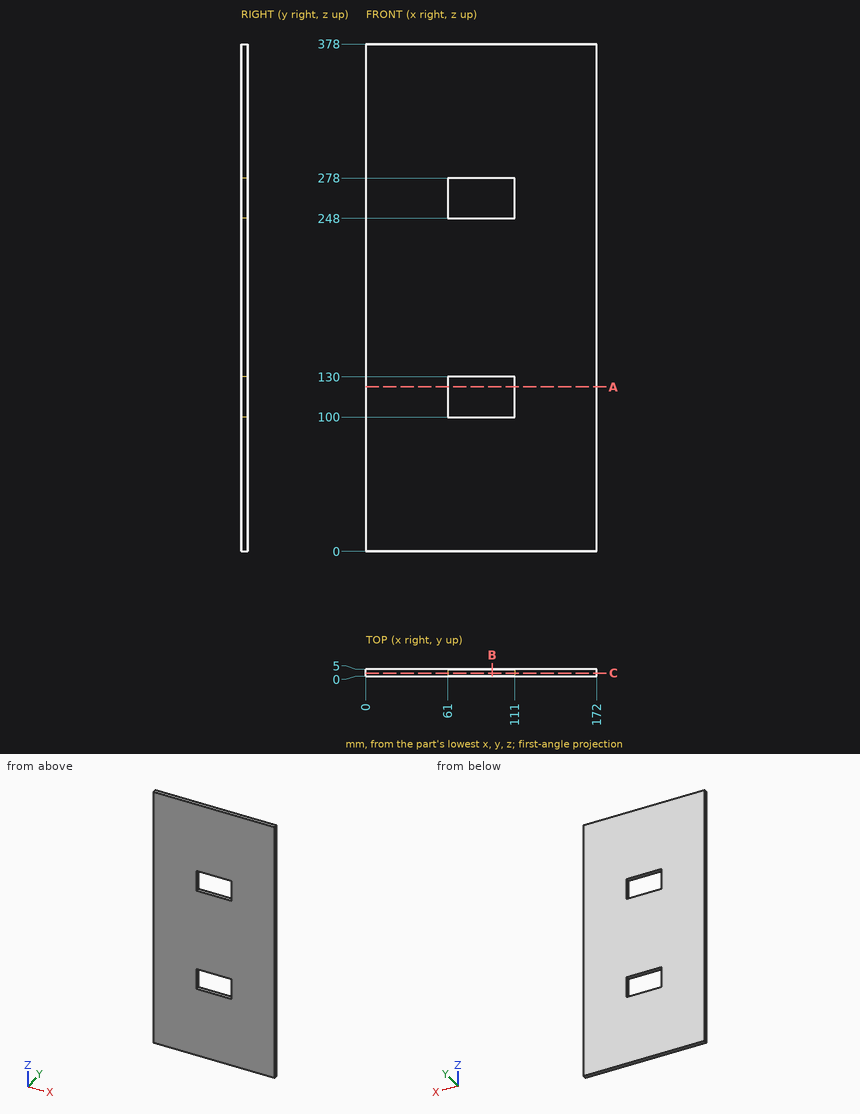
Source: three-view drawing plus pictorial views. Frame: mm from the lowest corner of the part. Round coordinates to 2 decimals unless told otherwise and drop trailing zeros. Order: outer loops, then holes, each group sorted by start corner. A loop starts at its lowest first (then second) coordinate and runs counter-clockwise, first axis right, second up. Notation, with made-up numbers: M 30,-6.5 L 89,-6.5 A28 ccw 89,22.5 Z; hole C -38,31 d1. An arc over 180 degrees is marked long. One line per item, written item: value.
(1) Pin query (flat end, axial travel): P1, Ø1.5, axis at x = 35.5, y = 2, coming from the -Z side. Return the tip coordinate at first contact, or that it passes through.
Result sheet:
P1: z = 0
(2) Cut plane B-B (x = 94). Return the cut outline in (y, z).
Result sheet:
outline: M 0,0 L 5,0 L 5,100 L 0,100 Z; M 0,130 L 5,130 L 5,248 L 0,248 Z; M 0,278 L 5,278 L 5,378 L 0,378 Z
(3) Cut plane A-A (z = 122.5). Return the cut outline in (x, y).
Result sheet:
outline: M 0,0 L 61,0 L 61,5 L 0,5 Z; M 111,0 L 172,0 L 172,5 L 111,5 Z
(4) Cut plane C-C (y = 2.2). Return the cut outline in (x, z).
Result sheet:
outline: M 0,0 L 172,0 L 172,378 L 0,378 Z; hole M 61,100 L 111,100 L 111,130 L 61,130 Z; hole M 61,248 L 111,248 L 111,278 L 61,278 Z
(5) Line query: probe 1 along Z at (x, y) = (98.5, 4); probe 2 along X at (y, z) = (3.55, 102). Output: solid intervals per line, ascending. Write a range as [from, to].
Result sheet:
probe 1: [0, 100], [130, 248], [278, 378]
probe 2: [0, 61], [111, 172]
